Source: CAD feature listing. Evaluate the final solid. Frame: model axes, mm. Face numbers are marked on the shaded views. A direction names the side the tool comes from. Give positions to 0.01 mm unless a question says otherwise; leave off trailing zeros. Order: outer loops, then holes, each group sorted by start corner. A loop starts at its lowest first (then second) coordinate and runs counter-clockwise, first axis right, second up. Notation, with made-up numbers: (68.5, 23.5) -> (82.5, 23.5) arc R26 ccw to (82.5, 45.5) -> close; hole circle Ø11 at (35.5, -38). An arc over 180 degrees is marked (long way). Answer in a Markdown table with one row per item.
```python
from build123d import *

# Parameters (mm, degrees)
SKETCH1_R           = 1.6
BOSS_EXTRUDE1_DEPTH = 3
SKETCH2_R           = 2.852011264
BOSS_EXTRUDE2_DEPTH = 1
SKETCH3_R           = 12
BOSS_EXTRUDE3_DEPTH = 17
SKETCH4_R           = 2.5
BOSS_EXTRUDE4_DEPTH = 16
FILLET1_R           = 3


with BuildPart() as part:
    # Sketch1 → Boss-Extrude1 (new body)
    with BuildSketch(Plane.XY):
        with BuildLine():
            Line((-71.781745931, -74.781745931), (-67.281745931, -74.781745931))
            ThreePointArc((-67.281745931, -74.781745931), (-65.867532368, -75.367532368), (-65.281745931, -76.781745931))
            Line((-65.281745931, -76.781745931), (-65.281745931, -78.781745931))
            ThreePointArc((-65.281745931, -78.781745931), (-65.867532368, -80.195959493), (-67.281745931, -80.781745931))
            Line((-67.281745931, -80.781745931), (-71.781745931, -80.781745931))
            ThreePointArc((-71.781745931, -80.781745931), (-73.903066274, -81.660425587), (-74.781745931, -83.781745931))
            Line((-74.781745931, -83.781745931), (-74.781745931, -88.281745931))
            ThreePointArc((-74.781745931, -88.281745931), (-75.367532368, -89.695959493), (-76.781745931, -90.281745931))
            Line((-76.781745931, -90.281745931), (-78.781745931, -90.281745931))
            ThreePointArc((-78.781745931, -90.281745931), (-80.195959493, -89.695959493), (-80.781745931, -88.281745931))
            Line((-80.781745931, -88.281745931), (-80.781745931, -83.781745931))
            ThreePointArc((-80.781745931, -83.781745931), (-81.660425587, -81.660425587), (-83.781745931, -80.781745931))
            Line((-83.781745931, -80.781745931), (-88.281745931, -80.781745931))
            ThreePointArc((-88.281745931, -80.781745931), (-89.695959493, -80.195959493), (-90.281745931, -78.781745931))
            Line((-90.281745931, -78.781745931), (-90.281745931, -76.781745931))
            ThreePointArc((-90.281745931, -76.781745931), (-89.695959493, -75.367532368), (-88.281745931, -74.781745931))
            Line((-88.281745931, -74.781745931), (-83.781745931, -74.781745931))
            ThreePointArc((-83.781745931, -74.781745931), (-81.660425587, -73.903066274), (-80.781745931, -71.781745931))
            Line((-80.781745931, -71.781745931), (-80.781745931, -67.281745931))
            ThreePointArc((-80.781745931, -67.281745931), (-80.195959493, -65.867532368), (-78.781745931, -65.281745931))
            Line((-78.781745931, -65.281745931), (-76.781745931, -65.281745931))
            ThreePointArc((-76.781745931, -65.281745931), (-75.367532368, -65.867532368), (-74.781745931, -67.281745931))
            Line((-74.781745931, -67.281745931), (-74.781745931, -71.781745931))
            ThreePointArc((-74.781745931, -71.781745931), (-73.903066274, -73.903066274), (-71.781745931, -74.781745931))
        make_face()
        with Locations((-77.781745931, -68.281745931)):
            Circle(SKETCH1_R, mode=Mode.SUBTRACT)
        with Locations((-68.281745931, -77.781745931)):
            Circle(SKETCH1_R, mode=Mode.SUBTRACT)
        with Locations((-77.781745931, -87.281745931)):
            Circle(SKETCH1_R, mode=Mode.SUBTRACT)
        with Locations((-87.281745931, -77.781745931)):
            Circle(SKETCH1_R, mode=Mode.SUBTRACT)
    extrude(amount=BOSS_EXTRUDE1_DEPTH)

    # Sketch2 → Boss-Extrude2 (add)
    with BuildSketch(Plane.XY.offset(3)):
        with Locations((-77.781745931, -77.781745931)):
            Circle(SKETCH2_R)
    extrude(amount=BOSS_EXTRUDE2_DEPTH)

    # Sketch3 → Boss-Extrude3 (add)
    with BuildSketch(Plane.XY.offset(4)):
        with Locations((-77.781745931, -77.781745931)):
            Circle(SKETCH3_R)
    extrude(amount=BOSS_EXTRUDE3_DEPTH)

    # Sketch4 → Boss-Extrude4 (add)
    with BuildSketch(Plane.XY.offset(21)):
        with Locations((-77.781745931, -77.781745931)):
            Circle(SKETCH4_R)
    extrude(amount=BOSS_EXTRUDE4_DEPTH)

    # Fillet1
    fillet1_edges = [part.edges().sort_by_distance(p)[0] for p in [
        (-89.781745931, -77.781745931, 4),
        (-89.781745931, -77.781745931, 21),
    ]]
    fillet(fillet1_edges, radius=FILLET1_R)


solid = part.part
```
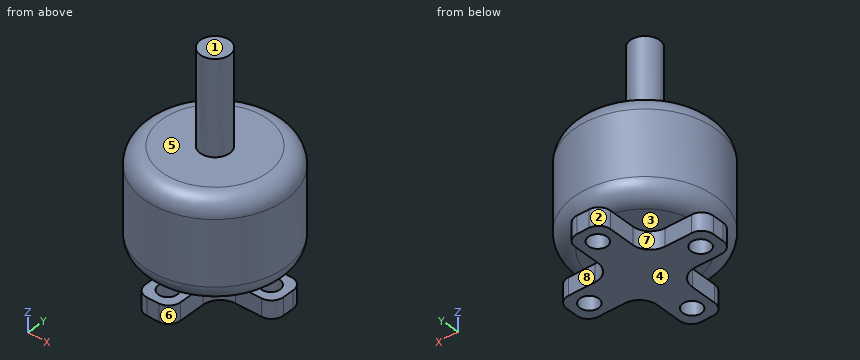
(1) Ray query, probe 1 along Z at (x, y) = (-73, -76.5); probe 2 along X at (y, z) = (-68.75, 17.5); probe 3 along Y at (x, z) = (-71.5, 2.5). Return the intervals inside material, ascending.
A:
| item | result |
|---|---|
| probe 1 | z = 0 to 3, 4 to 21 |
| probe 2 | x = -85.68 to -69.88 |
| probe 3 | y = -80.78 to -74.78 |
(2) Section query B-B (z = 22.5). Return the cut outline in (x, y).
A:
| item | result |
|---|---|
| outline | circle Ø5 at (-77.78, -77.78) |
(3) Section query D-D (z = 13.5). Return the cut outline in (x, y), plus the area to 3 significant figures.
A:
| item | result |
|---|---|
| outline | circle Ø24 at (-77.78, -77.78) |
| area | 452 mm^2 |
(4) Pull-direction query (Z, two-part tool) for the marked faces 1, 2 and 3; classes: +Z half, -Z half, draft (parallel to the pull), parting line (faces both ways), or undercut.
A:
| item | result |
|---|---|
| face 1 | +Z half |
| face 2 | draft |
| face 3 | undercut |
(5) First-contact query: pin 1 Ø12 at (y, z) = (-73.5, 29) entering from -X; pin 2 Ø1.5 at (y, z) = (-85.5, 1.5) entering from +X; pin 3 Ø0.9 at (y, z) = (-70.5, 1.5) entering from -X; pin 4 Ø12.5 at (x, y) = (-71.5, -74) entering from +Z. Flat tips, straight axial feed; report the tip coordinate or a pass-through.
A:
| item | result |
|---|---|
| pin 1 | stops at x = -80.28 |
| pin 2 | stops at x = -74.78 |
| pin 3 | stops at x = -80.78 |
| pin 4 | stops at z = 37 |
(6) Access query for the marked faces 4, 5, 6, 7 and 8. Directions: +Z, -Z, +X, -X, +Y, -Y. A direction counts if a zero-diameter tool reaches every point of the face in a straight line with its end or side. Return the directions, or none.
A:
| item | result |
|---|---|
| face 4 | -Z, +X, -X, +Y, -Y |
| face 5 | +Z |
| face 6 | -Z, +X, -Y |
| face 7 | -Z, -X, +Y |
| face 8 | -Z, +X, +Y |
(7) Section query A-A (x = -87.75). Give the number of separate pieces and of enclosed holes in the cut face, plus the area to 3 significant figures.
A:
| item | result |
|---|---|
| separate pieces | 3 |
| enclosed holes | 0 |
| area | 218 mm^2 |
